```python
from build123d import *

# Parameters (mm, degrees)
SKETCH1_W                    = 40
SKETCH1_H                    = 50
BASE_FLANGE1_DEPTH           = 2
EDGE_FLANGE1_STRIP_W         = 9.4732
EDGE_FLANGE1_STRIP_H         = 2
EDGE_FLANGE1_STRIP_CUT_DEPTH = 40
EDGE_FLANGE1_DEPTH           = 40
CUT_EXTRUDE1_REACH           = 51.689
SKETCH9_R                    = 1.4
SKETCH9_R_2                  = 4
CUT_EXTRUDE2_REACH           = 69.082
SKETCH11_R                   = 1.6
FILLET1_R                    = 10


# Sheet-metal steps are written as plain solids
with BuildPart() as part:
    # Sketch1 → Base-Flange1 (new body)
    with BuildSketch(Plane.XY):
        Rectangle(SKETCH1_W, SKETCH1_H)
    extrude(amount=-BASE_FLANGE1_DEPTH)

    # Edge-Flange1 strip (across the edge) → Edge-Flange1 strip cut (cut)
    with BuildSketch(Plane(origin=(20, -25, -2), x_dir=(0, 1, 0), z_dir=(-1, 0, 0))):
        with Locations((-2, -1)):
            Rectangle(EDGE_FLANGE1_STRIP_W, EDGE_FLANGE1_STRIP_H)
    extrude(amount=EDGE_FLANGE1_STRIP_CUT_DEPTH, mode=Mode.SUBTRACT)

    # Edge-Flange1 section (across the edge) → Edge-Flange1 (add)
    with BuildSketch(Plane(origin=(20, -25, -2), x_dir=(0, 1, 0), z_dir=(-1, 0, 0))):
        with BuildLine():
            Line((0, 0.7366), (0, 38))
            Line((0, 38), (2, 38))
            Line((2, 38), (2, 0.7366))
            ThreePointArc((2, 0.7366), (2.215745145, 0.215745145), (2.7366, 0))
            Line((2.7366, 0), (2.7366, -2))
            ThreePointArc((2.7366, -2), (0.801531583, -1.198468417), (0, 0.7366))
        make_face()
    extrude(amount=EDGE_FLANGE1_DEPTH)

    # Sketch9 → Cut-Extrude1 (cut, up to next)
    with BuildSketch(Plane(origin=(0, 0, -2), x_dir=(-1, 0, 0), z_dir=(0, 0, -1)), mode=Mode.PRIVATE) as cut_extrude1_sk1:
        with Locations((-15.5, 15.5)):
            Circle(SKETCH9_R)
    cut_extrude1_tool1 = extrude(cut_extrude1_sk1.sketch, amount=-CUT_EXTRUDE1_REACH, mode=Mode.PRIVATE) & part.part
    # Sketch9 → Cut-Extrude1 (cut, up to next)
    with BuildSketch(Plane(origin=(0, 0, -2), x_dir=(-1, 0, 0), z_dir=(0, 0, -1)), mode=Mode.PRIVATE) as cut_extrude1_sk2:
        with Locations((15.5, 15.5)):
            Circle(SKETCH9_R)
    cut_extrude1_tool2 = extrude(cut_extrude1_sk2.sketch, amount=-CUT_EXTRUDE1_REACH, mode=Mode.PRIVATE) & part.part
    # Sketch9 → Cut-Extrude1 (cut, up to next)
    with BuildSketch(Plane(origin=(0, 0, -2), x_dir=(-1, 0, 0), z_dir=(0, 0, -1)), mode=Mode.PRIVATE) as cut_extrude1_sk3:
        with Locations((15.5, -15.5)):
            Circle(SKETCH9_R)
    cut_extrude1_tool3 = extrude(cut_extrude1_sk3.sketch, amount=-CUT_EXTRUDE1_REACH, mode=Mode.PRIVATE) & part.part
    # Sketch9 → Cut-Extrude1 (cut, up to next)
    with BuildSketch(Plane(origin=(0, 0, -2), x_dir=(-1, 0, 0), z_dir=(0, 0, -1)), mode=Mode.PRIVATE) as cut_extrude1_sk4:
        with Locations((-15.5, -15.5)):
            Circle(SKETCH9_R)
    cut_extrude1_tool4 = extrude(cut_extrude1_sk4.sketch, amount=-CUT_EXTRUDE1_REACH, mode=Mode.PRIVATE) & part.part
    # Sketch9 → Cut-Extrude1 (cut, up to next)
    with BuildSketch(Plane(origin=(0, 0, -2), x_dir=(-1, 0, 0), z_dir=(0, 0, -1)), mode=Mode.PRIVATE) as cut_extrude1_sk5:
        Circle(SKETCH9_R_2)
    cut_extrude1_tool5 = extrude(cut_extrude1_sk5.sketch, amount=-CUT_EXTRUDE1_REACH, mode=Mode.PRIVATE) & part.part
    add(cut_extrude1_tool1.solids().sort_by_distance((15.5, 15.5, -2))[0], mode=Mode.SUBTRACT)
    add(cut_extrude1_tool2.solids().sort_by_distance((-15.5, 15.5, -2))[0], mode=Mode.SUBTRACT)
    add(cut_extrude1_tool3.solids().sort_by_distance((-15.5, -15.5, -2))[0], mode=Mode.SUBTRACT)
    add(cut_extrude1_tool4.solids().sort_by_distance((15.5, -15.5, -2))[0], mode=Mode.SUBTRACT)
    add(cut_extrude1_tool5.solids().sort_by_distance((0, 0, -2))[0], mode=Mode.SUBTRACT)

    # Sketch11 → Cut-Extrude2 (cut, up to next)
    with BuildSketch(Plane.XZ.offset(25), mode=Mode.PRIVATE) as cut_extrude2_sk1:
        with Locations(Location((-10, -21.3683, 0), (0, 0, 270))):
            Circle(SKETCH11_R)
    cut_extrude2_tool1 = extrude(cut_extrude2_sk1.sketch, amount=-CUT_EXTRUDE2_REACH, mode=Mode.PRIVATE) & part.part
    # Sketch11 → Cut-Extrude2 (cut, up to next)
    with BuildSketch(Plane.XZ.offset(25), mode=Mode.PRIVATE) as cut_extrude2_sk2:
        with Locations(Location((10, -21.3683, 0), (0, 0, 270))):
            Circle(SKETCH11_R)
    cut_extrude2_tool2 = extrude(cut_extrude2_sk2.sketch, amount=-CUT_EXTRUDE2_REACH, mode=Mode.PRIVATE) & part.part
    add(cut_extrude2_tool1.solids().sort_by_distance((-10, -25, -21.3683))[0], mode=Mode.SUBTRACT)
    add(cut_extrude2_tool2.solids().sort_by_distance((10, -25, -21.3683))[0], mode=Mode.SUBTRACT)

    # Fillet1
    fillet1_edges = [part.edges().sort_by_distance(p)[0] for p in [
        (20, -24, -40),
        (-20, -24, -40),
        (-20, 25, -1),
        (20, 25, -1),
    ]]
    fillet(fillet1_edges, radius=FILLET1_R)


solid = part.part
```
Check sheet for the modelled part. Datum: model origin and axes. Units: mm. Coordinates: 2 decimals unless noted, no trailing zeros. Order: outer loops, then holes, each group sorted by start corner. A loop starts at its lowest first (then second) coordinate and runs counter-clockwise, first axis right, second up. Notation, with made-up numbers: M -8,37.25 L 18,37.25 A32 cw 18,67.25 Z; hole C 65,86 d3. An arc over 180 degrees is marked long. Write each question's results on one line, items separated by ' | '. Start each with the question number.
1. Material ranges on probe 1 along Y at (x, z) = (15, -1); probe 2 along Y at (x, z) = (15.5, -0.7); probe 3 along Z at (x, y) = (13, 10), recorded low to high.
2. Mould release check, pull along X, two halves, no side actions. Record for faces 1 (the face through (4, 2, -2)), 2 (the face through (-17.15, -23.99, -36.99)), 3 (the face through (0.867, -3.905, -1.014)): +X half, -X half, draft (parallel to the pull), parting line (faces both ways), or undercut.
3. Cross-section at C-C on y = -15.5. Record the cut outline in (x, z).
4. Cross-section at B-B on y = 0. Record the cut outline in (x, z).
5. Cross-section at D-D on x = -6.5. Record the cut outline in (y, z).
6. Go/stop test with flat-tipped pins: P1, Ø8, axis at x = 15.5, y = -3, coming from the -Z side; P2, Ø5, axis at x = -3.5, z = -24.5, coming from the +Y side. Record where each tip stops, or that it passes through.
7. Cross-section at A-A on x = 0. Record the cut outline in (y, z).
Checks:
1) probe 1: y = -24.38 to -16.81, -14.19 to 14.19, 16.81 to 23.66 | probe 2: y = -24.09 to -16.9, -14.1 to 14.1, 16.9 to 23.35 | probe 3: z = -2 to 0
2) face 1: draft | face 2: -X half | face 3: undercut
3) outline: M -20,-2 L -16.9,-2 L -16.9,0 L -20,0 Z; M -14.1,-2 L 14.1,-2 L 14.1,0 L -14.1,0 Z; M 16.9,-2 L 20,-2 L 20,0 L 16.9,0 Z
4) outline: M -20,-2 L -4,-2 L -4,0 L -20,0 Z; M 4,-2 L 20,-2 L 20,0 L 4,0 Z
5) outline: M -25,-40 L -23,-40 L -23,-2.74 A0.74 cw -22.26,-2 L 25,-2 L 25,0 L -22.26,0 A2.74 ccw -25,-2.74 Z
6) P1: stops at z = -2 | P2: stops at y = -23
7) outline: M -25,-40 L -23,-40 L -23,-2.74 A0.74 cw -22.26,-2 L -4,-2 L -4,0 L -22.26,0 A2.74 ccw -25,-2.74 Z; M 4,-2 L 25,-2 L 25,0 L 4,0 Z
